Could you check a few things on this model? Use its own coordinates, in mm. Face numbers are marked on the shaded views. A direction names the side the tool comes from. Round coordinates to 2 decimals unless told otherwise and drop trailing zeros. Loops run counter-clockwise (first coordinate to the right, second up) from the corner with the lowest first, then second, coordinate; pieces in that order, holes last. Notation, with made-up numbers: (36, -32.75) - (79, -32.75) arc R19 ccw to (79, -5.75) - close; hole circle Ø8 at (73, 13.5). An arc over 180 degrees is marked (long way). Answer as CSV lines item,"result". Start each with the question number.
1) Which directions (+Z, -Z, +X, -X, +Y, -Y) give clear straight access to the entire face, cutting with the end or side of a thin tool? Please do the marked faces 1, 2, 3 and 4.
2) Suppose I cut it at C-C, the plane x = 5.25. Write out the boundary of the cut face in (y, z).
3) Please list where these lines run through material, in increasing order: line 1 along X through (y, z) = (7.5, 3.5); line 2 along X through (y, z) = (-8.75, 6.5); line 3 along Z through (x, y) = (-6.5, -6).
4) Suppose I cut it at D-D, the plane y = 3.5. Write out the boundary of the cut face in (x, z).
5) I'm going to push flat-ended pins straight in: pin 1 Ø4 at (x, z) = (9, 7.5) entering from -Y; pin 2 Ø4.5 at (x, y) = (5.5, 1) entering from -Z; pin 3 Ø0.9 at (x, y) = (-3.5, -8) entering from -Z. Where does each tip first touch, or does it pass through?
6) Suppose I cut it at B-B, the plane y = 0. Write out the boundary of the cut face in (x, z).
7) We'd pull the mould along X, two halves only. Please class the marked faces 5, 6 and 7: pulls with the +X half, pulls with the -X half, needs draft (parallel to the pull), parting line crosses it, or undercut.
```python
from build123d import *

# Parameters (mm, degrees)
BOSS_EXTRUDE1_DEPTH             = 6
BOSS_EXTRUDE1_2_DEPTH           = 6
CUT_EXTRUDE1_DEPTH              = 4
BOSS_EXTRUDE2_DEPTH             = 0.5
BOSS_EXTRUDE2_DEPTH_BACK        = 2
BOSS_EXTRUDE3_REACH             = 22.017
BOSS_EXTRUDE3_START             = -3
SKETCH6_R                       = 7.75
CUT_EXTRUDE2_DEPTH              = 17.227295759
FILLET1_R                       = 2
BOSS_EXTRUDE4_START             = 1.8
BOSS_EXTRUDE4_DEPTH             = 1.8
CUT_EXTRUDE3_DEPTH              = 2
BOSS_EXTRUDE5_DEPTH             = 3
CUT_EXTRUDE4_REACH              = 33.204
CUT_EXTRUDE4_END_RADIUS         = 7.75
SKETCH11_R                      = 3.1
BOSS_EXTRUDE6_DEPTH             = 8.3
TAP_DRILL_FOR_M2X0_4_TAP1_D     = 1.6
TAP_DRILL_FOR_M2X0_4_TAP1_DEPTH = 5
TAP_DRILL_FOR_M2X0_4_TAP1_TIP   = 0.480688495
FILLET2_R                       = 0.5


with BuildPart() as part:
    # Sketch1 → Boss-Extrude1 (new body)
    with BuildSketch(Plane.XY):
        Polygon((-8.605017992, 0), (-6.084666575, 6.084666575), (0, 8.605017992), (6.084666575, 6.084666575), (8.605017992, 0), (6.084666575, -6.084666575), (0, -8.605017992), (-6.084666575, -6.084666575), align=None)
    extrude(amount=BOSS_EXTRUDE1_DEPTH)

    # Sketch3 → Cut-Extrude1 (cut)
    with BuildSketch(Plane(origin=(0, 0, 0), x_dir=(-1, 0, 0), z_dir=(0, 0, -1))):
        Polygon((6.084666575, 6.084666575), (0, 8.605017992), (-6.084666575, 6.084666575), (-8.605017992, 0), (-6.084666575, -6.084666575), (0, -8.605017992), (6.084666575, -6.084666575), (8.605017992, 0), align=None)
    extrude(amount=-CUT_EXTRUDE1_DEPTH, mode=Mode.SUBTRACT)



with BuildPart() as body_2:
    # Sketch1 → Boss-Extrude1 2 (new body)
    with BuildSketch(Plane.XY):
        Polygon((-11.120367073, 0), (-7.863286966, 7.863286966), (0, 11.120367073), (7.863286966, 7.863286966), (11.120367073, 0), (7.863286966, -7.863286966), (0, -11.120367073), (-7.863286966, -7.863286966), align=None)
        Polygon((-7.097920102, 7.097920102), (0, 10.037974872), (7.097920102, 7.097920102), (10.037974872, 0), (7.097920102, -7.097920102), (0, -10.037974872), (-7.097920102, -7.097920102), (-10.037974872, 0), align=None, mode=Mode.SUBTRACT)
    extrude(amount=BOSS_EXTRUDE1_2_DEPTH)


with BuildPart() as part_1:
    add(part.part)

    add(body_2.part)  # Boss-Extrude2 merges body 2
    # Sketch4 → Boss-Extrude2 (add, two sides: drawn at the far end of the back side and taken through both)
    with BuildSketch(Plane.XY.offset(6).offset(-BOSS_EXTRUDE2_DEPTH_BACK)):
        Polygon((-11.120367073, 0), (-7.863286966, -7.863286966), (0, -11.120367073), (7.863286966, -7.863286966), (11.120367073, 0), (7.863286966, 7.863286966), (0, 11.120367073), (-7.863286966, 7.863286966), align=None)
    extrude(amount=BOSS_EXTRUDE2_DEPTH + BOSS_EXTRUDE2_DEPTH_BACK)

    # Sketch5 → Boss-Extrude3 (add, up to next)
    with BuildSketch(Plane(origin=(0, 0, 0), x_dir=(-1, 0, 0), z_dir=(0, 0, -1)).offset(BOSS_EXTRUDE3_START), mode=Mode.PRIVATE) as boss_extrude3_sk1:
        Polygon((-7.691079422, 5.665906826), (-9.451423211, 1.416060977), (-8.435155725, 0.995109201), (-6.674811936, 5.244955051), align=None)
    boss_extrude3_tool1 = extrude(boss_extrude3_sk1.sketch, amount=-BOSS_EXTRUDE3_REACH, mode=Mode.PRIVATE) - part_1.part
    # Sketch5 → Boss-Extrude3 (add, up to next)
    with BuildSketch(Plane(origin=(0, 0, 0), x_dir=(-1, 0, 0), z_dir=(0, 0, -1)).offset(BOSS_EXTRUDE3_START), mode=Mode.PRIVATE) as boss_extrude3_sk2:
        Polygon((1.416060977, -9.451423211), (5.665906826, -7.691079422), (5.244955051, -6.674811936), (0.995109201, -8.435155725), align=None)
    boss_extrude3_tool2 = extrude(boss_extrude3_sk2.sketch, amount=-BOSS_EXTRUDE3_REACH, mode=Mode.PRIVATE) - part_1.part
    add(boss_extrude3_tool1.solids().sort_by_distance((8.063118, 3.330508, 3))[0])
    add(boss_extrude3_tool2.solids().sort_by_distance((-3.330508, -8.063118, 3))[0])

    # Sketch6 → Cut-Extrude2 (cut, through all)
    with BuildSketch(Plane(origin=(0, 0, 4), x_dir=(-1, 0, 0), z_dir=(0, 0, -1))):
        Circle(SKETCH6_R)
    extrude(amount=-CUT_EXTRUDE2_DEPTH, mode=Mode.SUBTRACT)

    # Fillet1
    fillet1_edges = [part_1.edges().sort_by_distance(p)[0] for p in [
        (-7.863286966, -7.863286966, 3.25),
        (0, -11.120367073, 3.25),
        (7.863286966, -7.863286966, 3.25),
        (11.120367073, 0, 3.25),
        (7.863286966, 7.863286966, 3.25),
        (0, 11.120367073, 3.25),
        (-7.863286966, 7.863286966, 3.25),
        (-11.120367073, 0, 3.25),
        (7.097920102, 7.097920102, 2),
        (0, 10.037974872, 2),
        (10.037974872, 0, 2),
        (7.097920102, -7.097920102, 2),
        (0, -10.037974872, 2),
        (-7.097920102, -7.097920102, 2),
        (-10.037974872, 0, 2),
        (-7.097920102, 7.097920102, 2),
    ]]
    fillet(fillet1_edges, radius=FILLET1_R)

    # Sketch9 → Boss-Extrude4 (add)
    with BuildSketch(Plane.XY.offset(6.5).offset(BOSS_EXTRUDE4_START)):
        with BuildLine():
            ThreePointArc((8.180312302, 7.097920102), (7.746766799, 7.746766799), (7.097920102, 8.180312302))
            Line((7.097920102, 8.180312302), (0.765366865, 10.803341737))
            ThreePointArc((0.765366865, 10.803341737), (0, 10.955582672), (-0.765366865, 10.803341737))
            Line((-0.765366865, 10.803341737), (-6.694671234, 8.347343452))
            Line((-6.694671234, 8.347343452), (-3.924480161, 7.19989274))
            ThreePointArc((-3.924480161, 7.19989274), (7.575812167, -3.138004145), (-7.866119515, -2.316066445))
            Line((-7.866119515, -2.316066445), (-10.636310587, -1.168615733))
            Line((-10.636310587, -1.168615733), (-8.180312302, -7.097920102))
            ThreePointArc((-8.180312302, -7.097920102), (-7.746766799, -7.746766799), (-7.097920102, -8.180312302))
            Line((-7.097920102, -8.180312302), (-0.765366865, -10.803341737))
            ThreePointArc((-0.765366865, -10.803341737), (0, -10.955582672), (0.765366865, -10.803341737))
            Line((0.765366865, -10.803341737), (7.097920102, -8.180312302))
            ThreePointArc((7.097920102, -8.180312302), (7.746766799, -7.746766799), (8.180312302, -7.097920102))
            Line((8.180312302, -7.097920102), (10.803341737, -0.765366865))
            ThreePointArc((10.803341737, -0.765366865), (10.955582672, 0), (10.803341737, 0.765366865))
            Line((10.803341737, 0.765366865), (8.180312302, 7.097920102))
        make_face()
    extrude(amount=-BOSS_EXTRUDE4_DEPTH)

    # Sketch10 → Cut-Extrude3 (cut)
    with BuildSketch(Plane.XY.offset(6.5)):
        Polygon((-8.848789177, 8.806651439), (-3.151903136, 6.446923978), (-6.787395744, -2.329931581), (-12.484281785, 0.02979588), align=None)
    extrude(amount=-CUT_EXTRUDE3_DEPTH, mode=Mode.SUBTRACT)

    # Sketch12 → Boss-Extrude5 (add)
    with BuildSketch(Plane.XY.offset(8.3)):
        with BuildLine():
            Line((0, -10.955582672), (12.107294918, -10.42696676))
            Line((12.107294918, -10.42696676), (15.934129241, -1.188171435))
            Line((15.934129241, -1.188171435), (7.746766799, 7.746766799))
            Line((7.746766799, 7.746766799), (7.287962899, 6.639116202))
            Line((7.287962899, 6.639116202), (9.879462205, 0.382683432))
            ThreePointArc((9.879462205, 0.382683432), (9.955582672, 0), (9.879462205, -0.382683432))
            Line((9.879462205, -0.382683432), (7.256432769, -6.715236669))
            ThreePointArc((7.256432769, -6.715236669), (7.039660018, -7.039660018), (6.715236669, -7.256432769))
            Line((6.715236669, -7.256432769), (0.4588039, -9.847932075))
            Line((0.4588039, -9.847932075), (0, -10.955582672))
        make_face()
    extrude(amount=-BOSS_EXTRUDE5_DEPTH)

    # Cut-Extrude4: up to this cylinder (the profile starts outside it)
    cut_extrude4_end = Plane(origin=(0, 0, 9.5), z_dir=(0, 0, -1)) * Cylinder(CUT_EXTRUDE4_END_RADIUS, 82.908, mode=Mode.PRIVATE)
    # Sketch11 → Cut-Extrude4 (cut, up to the surface)
    with BuildSketch(Plane(origin=(14.020712079, -5.807569097, 0), x_dir=(0, 0, -1), z_dir=(0.9238795325112878, -0.38268343236508723, 0)), mode=Mode.PRIVATE) as cut_extrude4_sk1:
        with Locations((-9.5, 0)):
            Circle(SKETCH11_R)
    cut_extrude4_tool1 = extrude(cut_extrude4_sk1.sketch, amount=-CUT_EXTRUDE4_REACH, mode=Mode.PRIVATE) - cut_extrude4_end
    add(cut_extrude4_tool1.solids().sort_by_distance((14.020712, -5.807569, 9.5))[0], mode=Mode.SUBTRACT)

    # Sketch13 → Boss-Extrude6 (add)
    with BuildSketch(Plane.XY.offset(8.3)):
        with BuildLine():
            Line((-8.180312302, -7.097920102), (-7.001403735, -9.944057152))
            ThreePointArc((-7.001403735, -9.944057152), (-6.228243887, -10.865473179), (-5.066405895, -11.176786731))
            Line((-5.066405895, -11.176786731), (0.174311485, -10.947972068))
            Line((0.174311485, -10.947972068), (-8.180312302, -7.097920102))
        make_face()
        with BuildLine():
            Line((7.864642123, 7.618128456), (4.320691724, 11.485671654))
            ThreePointArc((4.320691724, 11.485671654), (3.279016278, 12.087083253), (2.080770186, 11.982250304))
            Line((2.080770186, 11.982250304), (-0.765366865, 10.803341737))
            Line((-0.765366865, 10.803341737), (7.864642123, 7.618128456))
        make_face()
    extrude(amount=-BOSS_EXTRUDE6_DEPTH)

    # Tap Drill for M2x0.4 Tap1
    with Locations(Plane.XY.offset(8.3)):
        with Locations((-5.235070699, -8.98020238), (2.648208008, 10.05171599)):
            Hole(TAP_DRILL_FOR_M2X0_4_TAP1_D / 2, depth=TAP_DRILL_FOR_M2X0_4_TAP1_DEPTH)
            with Locations((0, 0, -(TAP_DRILL_FOR_M2X0_4_TAP1_DEPTH + TAP_DRILL_FOR_M2X0_4_TAP1_TIP / 2))):  # 118° drill point
                Cone(0, TAP_DRILL_FOR_M2X0_4_TAP1_D / 2, TAP_DRILL_FOR_M2X0_4_TAP1_TIP, mode=Mode.SUBTRACT)

    # Fillet2
    fillet2_edges = [part_1.edges().sort_by_distance(p)[0] for p in [
        (9.451423211, 1.416060977, 3.5),
        (7.691079422, 5.665906826, 3.5),
        (-5.665906826, -7.691079422, 3.5),
        (-1.416060977, -9.451423211, 3.5),
    ]]
    fillet(fillet2_edges, radius=FILLET2_R)


solid = part_1.part
```
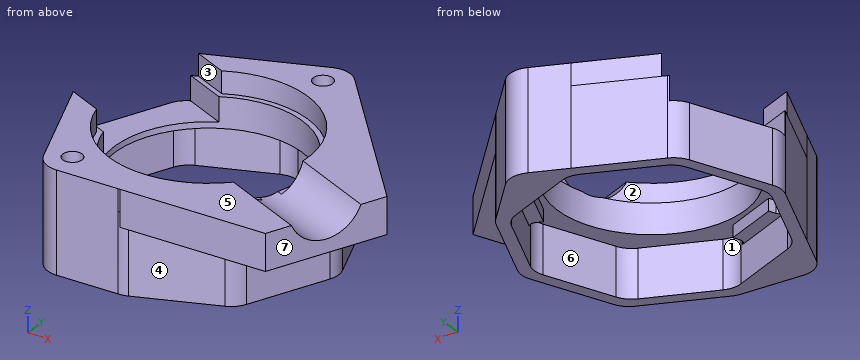
Filled sheet:
1,face 1,"-Z"
1,face 2,"+Z"
1,face 3,"+Z, -X"
1,face 4,"-Z, +X, -Y"
2,outline,"(-10.73, 5.3) - (-8.95, 5.3) - (-8.95, 0) - (-7.86, 0) - (-7.86, 4) - (-5.7, 4) - (-5.7, 6.5) - (-6.3, 6.5) - (-6.3, 8.3) - (-10.73, 8.3) - close; (5.7, 4) - (7.86, 4) - (7.86, 0) - (10.47, 0) - (10.47, 8.3) - (6.3, 8.3) - (6.3, 6.5) - (5.7, 6.5) - close"
3,line 1,"-7.96 to -6.13, 6.13 to 7.96"
3,line 2,"-7.5 to -6, -4.47 to 12.8"
3,line 3,"4 to 8.3"
4,outline,"(-9.67, 0) - (-8.59, 0) - (-8.59, 4) - (-6.91, 4) - (-6.91, 4.5) - (-9.67, 4.5) - close; (6.91, 4) - (7.4, 4) - (7.4, 3) - (8.59, 3) - (8.59, 0) - (9.67, 0) - (9.67, 5.3) - (11.64, 5.3) - (11.64, 8.3) - (7.42, 8.3) - (7.42, 6.5) - (6.91, 6.5) - close"
5,pin 1,"y = -10.65"
5,pin 2,"z = 4"
5,pin 3,"z = 3"
6,outline,"(-10.96, 0) - (-9.87, 0) - (-9.87, 4) - (-7.75, 4) - (-7.75, 4.5) - (-10.96, 4.5) - close; (7.75, 4) - (9.87, 4) - (9.87, 0) - (10.96, 0) - (10.96, 5.3) - (14.85, 5.3) - (14.85, 8.3) - (8.2, 8.3) - (8.2, 6.5) - (7.75, 6.5) - close"
7,face 5,"needs draft"
7,face 6,"undercut"
7,face 7,"pulls with the +X half"
